CAD build for the part. Positions are in the model's coordinates, mm. Face numbers are marked on the shaded views. A direction names the side the tool comes from. Round coordinates to 2 decimals unless told otherwise and drop trailing zeros. Order: outer loops, then holes, each group sorted by start corner. A loop starts at its lowest first (then second) coordinate and runs counter-clockwise, first axis right, second up.
```python
from build123d import *

# Parameters (mm, degrees)
F0_R     = 8.5
F1_DEPTH = 25.4
F3_D     = 7.3
F5_DEPTH = 18.542
F6_R     = 7.2
F6_R_2   = 3.65
F7_DEPTH = 5.9


with BuildPart() as f1:
    # F0 (on Top) → F1 (new body)
    with BuildSketch(Plane.XY):
        Circle(F0_R)
    extrude(amount=F1_DEPTH)

    # F3 (through all)
    with Locations(Plane.XY.offset(25.4)):
        with Locations((0, 0)):
            Hole(F3_D / 2)

    # F4 (on face) → F5 (cut)
    with BuildSketch(Plane.XY.offset(25.4)):
        with BuildLine():
            Line((-3.65, 7.6764249492), (-3.65, 0))
            ThreePointArc((-3.65, 0), (0, 3.65), (3.65, 0))
            Line((3.65, 0), (3.65, 7.6764249492))
            ThreePointArc((3.65, 7.6764249492), (0, 8.5), (-3.65, 7.6764249492))
        make_face()
    extrude(amount=-F5_DEPTH, mode=Mode.SUBTRACT)

    # F6 (on face) → F7 (cut)
    with BuildSketch(Plane(origin=(0, 0, 0), x_dir=(1, 0, 0), z_dir=(0, 0, -1))):
        Circle(F6_R)
        Circle(F6_R_2, mode=Mode.SUBTRACT)
    extrude(amount=-F7_DEPTH, mode=Mode.SUBTRACT)


solid = f1.part
```
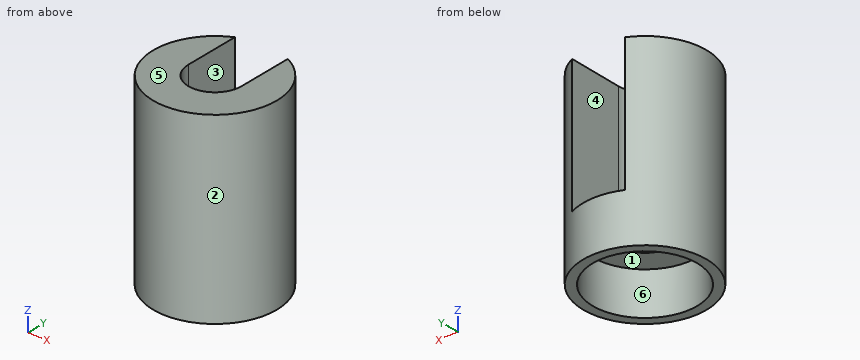
1. Pin check, flat tips, straight feed: P1, Ø1, axis at x = -1, y = 5, coming from the +Z side; P2, Ø6, axis at x = 0, y = 0, coming from the +Z side; P3, Ø4, axis at y = 5.5, z = 20, coming from the +X side; P4, Ø4, axis at x = -2.5, y = -2, coming from the -Z side. Stop position of each tip, or through.
2. Mould opens along Y. For the marked faces 1, 2 and 3 say: released by +Y, released by -Y, zero draft, split by the parting line, or undercut.
3. Drill centre lines: line 1 (Y direction, x = 0, z = 4.4); line 2 (X direction, y = 6.5, z = 5.5). Where is each one in solid material? Low to high.
4. Cut at A-A, the plane x = 0. Write the cut outline in (y, z).
5. Cut at C-C, the plane z = 5.25. Write the cut outline in (x, y).
6. Tool access for the marked faces 4, 5 and 6: list every direction of +Z, -Z, +X, -X, +Y, -Y with a clear straight run to the whole face (end or side of a thin tool).
7. Cut at B-B, the plane y = 2.5. Write the cut outline in (x, z).
8. Cut at D-D, the plane y = -6.75. Write the cut outline in (x, z), and give its area (3 significant figures).
Outcome:
1. P1: stops at z = 6.86
1. P2: passes through
1. P3: stops at x = 7.75
1. P4: stops at z = 5.9
2. face 1: undercut
2. face 2: split by the parting line
2. face 3: zero draft
3. line 1: y = -8.5 to -7.2, 7.2 to 8.5
3. line 2: x = -5.48 to -3.1, 3.1 to 5.48
4. outline: (-8.5, 0) - (-7.2, 0) - (-7.2, 5.9) - (-3.65, 5.9) - (-3.65, 25.4) - (-8.5, 25.4) - close; (3.65, 5.9) - (7.2, 5.9) - (7.2, 0) - (8.5, 0) - (8.5, 6.86) - (3.65, 6.86) - close
5. outline: circle Ø17 at (0, 0); hole circle Ø14.4 at (0, 0)
6. face 4: +Z, +Y
6. face 5: +Z, +X, -X, +Y, -Y
6. face 6: -Z
7. outline: (-8.12, 0) - (-6.75, 0) - (-6.75, 5.9) - (-2.66, 5.9) - (-2.66, 6.86) - (-3.65, 6.86) - (-3.65, 25.4) - (-8.12, 25.4) - close; (2.66, 5.9) - (6.75, 5.9) - (6.75, 0) - (8.12, 0) - (8.12, 25.4) - (3.65, 25.4) - (3.65, 6.86) - (2.66, 6.86) - close
8. outline: (-5.17, 0) - (-2.51, 0) - (-2.51, 5.9) - (2.51, 5.9) - (2.51, 0) - (5.17, 0) - (5.17, 25.4) - (-5.17, 25.4) - close
8. area: 233 mm2
